```python
from build123d import *

# Parameters (mm, degrees)
F0_R          = 7.5
F0_R_2        = 4
F1_DEPTH      = 8
F0_R_3        = 3
F2_DEPTH      = 8
F3_DEPTH      = 1
F3_DEPTH_BACK = 1


with BuildPart() as f1:
    # F0 (on Top) → F1 (new body)
    with BuildSketch(Plane.XY):
        Circle(F0_R)
        Circle(F0_R_2, mode=Mode.SUBTRACT)
    extrude(amount=F1_DEPTH)

    # F0 (on Top) → F2 (join)
    with BuildSketch(Plane.XY):
        Circle(F0_R)
        Circle(F0_R_2, mode=Mode.SUBTRACT)
        Circle(F0_R_2)
        Circle(F0_R_3, mode=Mode.SUBTRACT)
    extrude(amount=-F2_DEPTH)

    # F0 (on Top) → F3 (join, two sides)
    with BuildSketch(Plane.XY) as f3_sk:
        Circle(F0_R_2)
        Circle(F0_R_3, mode=Mode.SUBTRACT)
        Circle(F0_R_3)
    extrude(amount=F3_DEPTH)
    extrude(f3_sk.sketch, amount=-F3_DEPTH_BACK)


solid = f1.part
```
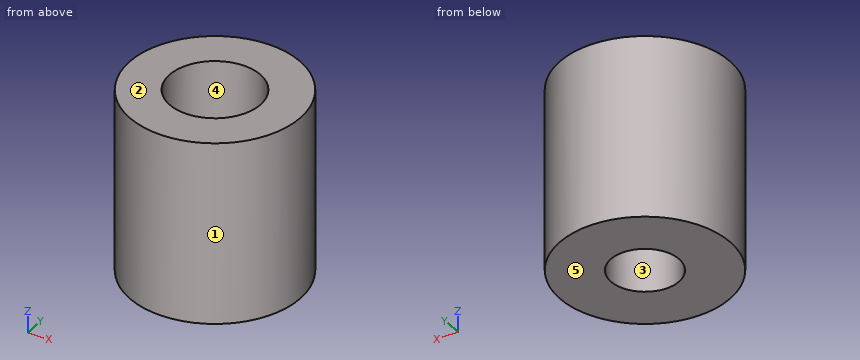
Geometry check sheet. Reference: the model listing, model coordinates, mm. Face numbers are marked on the shaded views. A direction names the side the tool comes from. Give positions to 0.01 mm unless a question says otherwise; leave off trailing zeros. Loops run counter-clockwise (first coordinate to the right, second up) from the corner with the lowest first, then second, coordinate; pieces in that order, holes last. Notation, with made-up numbers: M 89,80.25 L 122,80.25 A31 cw 122,115.25 Z; hole C -0.75,68.5 d7. An arc over 180 degrees is marked long. Write item = value, one per line. Start each with the question number.
1. Section check C-C, the plane z = -3.75. Enter the section's corners in (x, y).
2. Draft check along X on the marked faces 1, 2 and 3. Enter one of: +X half, -X half, draft (parallel to the pull), parting line (faces both ways), or undercut.
3. Section check D-D, the plane x = 3.75. Enter the section's corners in (y, z).
4. Go/stop test with flat-tipped pins: P1, Ø2, axis at y = 2, z = 0, coming from the -X side; P2, Ø2.5, axis at x = 0.5, y = 2, coming from the +Z side; P3, Ø6, axis at y = 4, z = -5.5, coming from the +X side. Record where each tip stops, or that it passes through.
5. Tool access check on the marked faces 4 and 5. Record the directions out of +Z, -Z, +X, -X, +Y, -Y that give a thin tool (end or side, any length) a straight path to the whole face; none if there is none.
6. Thickness scan on probe 1 along Y at (x, z) = (0, 3); probe 2 along Y at (x, z) = (0, -6); probe 3 along Z at (x, y) = (-1.75, 3.25). Record the ranges inside material, lowest first.
7. Section check A-A, the plane y = 0. Enter the section's corners in (x, z), plus the area to 3 significant figures.
Values follow:
q1.outline = C 0,0 d15; hole C 0,0 d6
q2.face_1 = parting line
q2.face_2 = draft
q2.face_3 = undercut
q3.outline = M -6.5,-8 L 6.5,-8 L 6.5,8 L 1.39,8 L 1.39,1 L -1.39,1 L -1.39,8 L -6.5,8 Z
q4.P1 = -7.43
q4.P2 = 1
q4.P3 = 7.43
q5.face_4 = +Z
q5.face_5 = -Z, +X, -X, +Y, -Y
q6.probe_1 = -7.5 to -4, 4 to 7.5
q6.probe_2 = -7.5 to -3, 3 to 7.5
q6.probe_3 = -8 to 1
q7.outline = M -7.5,-8 L -3,-8 L -3,-1 L 3,-1 L 3,-8 L 7.5,-8 L 7.5,8 L 4,8 L 4,1 L -4,1 L -4,8 L -7.5,8 Z
q7.area = 142 mm^2
